```python
from build123d import *

# Parameters (mm, degrees)
F0_R      = 12.5
F0_R_2    = 2.2070756532
F1_DEPTH  = 16
F2_W      = 30
F2_H      = 115
F2_W_2    = 115
F2_H_2    = 30
F3_DEPTH  = 30
F5_W      = 47.7929243468
F5_H      = 100
F5_W_2    = 30
F5_W_3    = 37.2070756532
F6_DEPTH  = 5
F7_W      = 115
F7_H      = 100
F8_DEPTH  = 5
F10_W     = 115
F10_H     = 100
F11_DEPTH = 5
F9_W      = 30
F9_H      = 100
F9_W_2    = 37.2870707512
F13_DEPTH = 5
F14_D     = 8
F14_DEPTH = 35.001


with BuildPart() as f1:
    # F0 (on Front) → F1 (new body)
    with BuildSketch(Plane.XZ):
        with BuildLine():
            Line((-699.9135494232, 64.4235223532), (-699.9135494232, -435.5764776468))
            Line((-699.9135494232, -435.5764776468), (-70.5764776468, -435.5764776468))
            Line((-70.5764776468, -435.5764776468), (0.0864505768, -364.9135494232))
            Line((0.0864505768, -364.9135494232), (0.0864505768, -2.20538188))
            ThreePointArc((0.0864505768, -2.20538188), (-2.2070756532, 0), (0.0864505768, 2.20538188))
            Line((0.0864505768, 2.20538188), (0.0864505768, 64.4235223532))
            Line((0.0864505768, 64.4235223532), (-149.9135494232, 64.4235223532))
            Line((-149.9135494232, 64.4235223532), (-149.9135494232, 49.4235223532))
            Line((-149.9135494232, 49.4235223532), (-319.9135494232, 49.4235223532))
            Line((-319.9135494232, 49.4235223532), (-319.9135494232, 64.4235223532))
            Line((-319.9135494232, 64.4235223532), (-699.9135494232, 64.4235223532))
        make_face()
        with Locations((-599.9135494232, -355.5764776468)):
            Circle(F0_R, mode=Mode.SUBTRACT)
        with Locations((-594.9135494232, -320.5764776468)):
            Circle(F0_R_2, mode=Mode.SUBTRACT)
        with Locations((-509.9135494232, -320.5764776468)):
            Circle(F0_R_2, mode=Mode.SUBTRACT)
        with Locations((-594.9135494232, -250.5764776468)):
            Circle(F0_R_2, mode=Mode.SUBTRACT)
        with Locations((-509.9135494232, -250.5764776468)):
            Circle(F0_R_2, mode=Mode.SUBTRACT)
        with Locations((-99.9135494232, -320.5764776468)):
            Circle(F0_R_2, mode=Mode.SUBTRACT)
        with Locations((-19.9135494232, -355.5764776468)):
            Circle(F0_R, mode=Mode.SUBTRACT)
        with Locations((-14.9135494232, -320.5764776468)):
            Circle(F0_R_2, mode=Mode.SUBTRACT)
        with Locations((-99.9135494232, -250.5764776468)):
            Circle(F0_R_2, mode=Mode.SUBTRACT)
        with Locations((-14.9135494232, -250.5764776468)):
            Circle(F0_R_2, mode=Mode.SUBTRACT)
        with Locations((-399.9135494232, -160.5764776468)):
            Circle(F0_R_2, mode=Mode.SUBTRACT)
        with Locations((-400.6345868111, -90.5764776468)):
            Circle(F0_R_2, mode=Mode.SUBTRACT)
        with Locations((-594.9135494232, -25.5764776468)):
            Circle(F0_R_2, mode=Mode.SUBTRACT)
        with Locations((-599.9135494232, 44.4235223532)):
            Circle(F0_R, mode=Mode.SUBTRACT)
        with Locations((-509.9135494232, -25.5764776468)):
            Circle(F0_R_2, mode=Mode.SUBTRACT)
        with Locations((-509.9135494232, 44.4235223532)):
            Circle(F0_R_2, mode=Mode.SUBTRACT)
        with Locations((-314.9135494232, -160.5764776468)):
            Circle(F0_R_2, mode=Mode.SUBTRACT)
        with Locations((-315.6345868111, -90.5764776468)):
            Circle(F0_R_2, mode=Mode.SUBTRACT)
        with Locations((-19.9135494232, 44.4235223532)):
            Circle(F0_R, mode=Mode.SUBTRACT)
        with BuildLine():
            ThreePointArc((0.0864505768, 2.20538188), (-2.2070756532, 0), (0.0864505768, -2.20538188))
            Line((0.0864505768, -2.20538188), (0.0864505768, 2.20538188))
        make_face()
        with BuildLine():
            Line((0.0864505768, 2.20538188), (0.0864505768, -2.20538188))
            ThreePointArc((0.0864505768, -2.20538188), (1.5909094729, -1.5297679523), (2.2070756532, 0))
            ThreePointArc((2.2070756532, 0), (1.5909094729, 1.5297679523), (0.0864505768, 2.20538188))
        make_face()
    extrude(amount=-F1_DEPTH)

    # F2 (on Front) → F3 (join)
    with BuildSketch(Plane.XZ):
        with Locations((-547.1206250764, -280.2835533)):
            Rectangle(F2_W, F2_H)
        with Locations((-355.6849062443, -120.1901584864)):
            Rectangle(F2_W, F2_H)
        with Locations((-547.2006201744, 6.2219314277)):
            Rectangle(F2_W, F2_H)
        with Locations((-62.3018592596, -282.930508256)):
            Rectangle(F2_W, F2_H)
        with Locations((-59.2683969438, -3.8263390213)):
            Rectangle(F2_W_2, F2_H_2)
    extrude(amount=F3_DEPTH)

    # F5 (on face) → F6 (join)
    with BuildSketch(Plane.XZ.offset(30)):
        with Locations((-586.0170872498, -285.5764776468)):
            Rectangle(F5_W, F5_H)
        with Locations((-547.1206250764, -285.5764776468)):
            Rectangle(F5_W_2, F5_H)
        with Locations((-513.5170872498, -285.5764776468)):
            Rectangle(F5_W_3, F5_H)
    extrude(amount=F6_DEPTH)

    # F7 (on face) → F8 (join)
    with BuildSketch(Plane.XZ.offset(30)):
        with Locations((-57.4135494232, -282.930508256)):
            Rectangle(F7_W, F7_H)
    extrude(amount=F8_DEPTH)

    # F10 (on face) → F11 (join)
    with BuildSketch(Plane.XZ.offset(30)):
        with Locations((-358.1345868111, -124.6901584864)):
            Rectangle(F10_W, F10_H)
    extrude(amount=F11_DEPTH)

    # F9 (on face) → F13 (join)
    with BuildSketch(Plane.XZ.offset(30)):
        Polygon((-562.2006201744, -40.5764776468), (-562.2006201744, 59.4235223532), (-574.9135494232, 59.4235223532), (-574.9135494232, 24.4235223532), (-609.9135494232, 24.4235223532), (-609.9135494232, -40.5764776468), align=None)
        with Locations((-547.2006201744, 9.4235223532)):
            Rectangle(F9_W, F9_H)
        with Locations((-513.5570847988, 9.4235223532)):
            Rectangle(F9_W_2, F9_H)
    extrude(amount=F13_DEPTH)

    # F14 (through all, one way)
    with BuildSketch(Plane(origin=(0, 0, 0), x_dir=(1, 0, 0), z_dir=(0, 1, 0))):
        with Locations((-594.9135494232, 250.5764776468), (-594.9135494232, 320.5764776468), (-509.9135494232, 320.5764776468), (-509.9135494232, 250.5764776468), (-400.6345868111, 90.5764776468), (-315.6345868111, 90.5764776468), (-399.9135494232, 160.5764776468), (-314.9135494232, 160.5764776468), (-594.9135494232, 25.5764776468), (-509.9135494232, 25.5764776468), (-509.9135494232, -44.4235223532), (-99.9135494232, 320.5764776468), (-99.9135494232, 250.5764776468), (-14.9135494232, 320.5764776468), (-14.9135494232, 250.5764776468)):
            Circle(F14_D / 2)
    extrude(amount=-F14_DEPTH, mode=Mode.SUBTRACT)


solid = f1.part
```
CAD build for the part. Positions are in the model's coordinates, mm. A direction names the side the tool comes from. Round coordinates to 2 decimals unless told otherwise and drop trailing zeros. Order: outer loops, then holes, each group sorted by start corner. A loop starts at its lowest first (then second) coordinate and runs counter-clockwise, first axis right, second up. Notation, with made-up numbers: (31, -37) - (55, -37) arc R35 cw to (55, -1) - close; hole circle Ø7 at (75, 77). An arc over 180 degrees is marked (long way). Use CSV: the item, a comma, the result in double quotes. Start each with the question number.
1) Saw through at D-D (z = -399). List the corners of the cut face in (x, y).
2) Wall check: L1, parallel to Y at x = -334, z = -132.5; L2, parallel to X at y = -15, z = -16; L3, parallel to Y at x = -433.5, z = -344. Give the ranges that are in metal, low to high. Write a range as [from, to].
3) Pin check, flat tips, straight feed: pin 1 Ø5 at (x, z) = (-400.63, -90.58) entering from -Y; pin 2 Ø5.5 at (x, y) = (-594, -32) entering from +Z; pin 3 Ø5.5 at (y, z) = (-32.5, -294) entering from -X. Stop position of each tip, or through.
4) Saw through at C-C (x = -205). List the corners of the cut face in (y, z).
5) Saw through at A-A (y = -7). List the corners of the cut face in (x, z).
6) Two-plate mould, pull along Y, no slides. Class faces 1 (the flat face through (-547, -15, -51.278)), 2 (the flat face through (-359, -35, -124)), 3 (the flat face through (-24, -30, -282)): pulls with the +Y half, pulls with the -Y half, needs draft (parallel to the pull), parting line crosses it, or undercut.
7) Tool access for faces 4 (the flat face through (-60, -30, -4)), 5 (the flat face through (-319.914, 8, 57)), 6 (the flat face through (-547, -15, 63.722)), 7 (the flat face through (-63, -15, -225.431)), 8 (the flat face through (-1.768, -15, -4)): list every direction of +Z, -Z, +X, -X, +Y, -Y with a clear straight run to the whole face (end or side of a thin tool).
8) Saw through at B-B (z = -105.5). List the corners of the cut face in (x, y).
Values follow:
1,outline,"(-699.91, 0) - (-34, 0) - (-34, 16) - (-699.91, 16) - close"
2,L1,"y = [-35, -30], [0, 16]"
2,L2,"x = [-562.2, -532.2], [-116.77, -1.77]"
2,L3,"y = [0, 16]"
3,pin 1,"stops at y = 0"
3,pin 2,"stops at z = 24.42"
3,pin 3,"stops at x = -609.91"
4,outline,"(0, -435.58) - (16, -435.58) - (16, 49.42) - (0, 49.42) - close"
5,outline,"(-562.2, -51.28) - (-532.2, -51.28) - (-532.2, 63.72) - (-562.2, 63.72) - close; (-562.12, -337.78) - (-532.12, -337.78) - (-532.12, -222.78) - (-562.12, -222.78) - close; (-370.68, -177.69) - (-340.68, -177.69) - (-340.68, -62.69) - (-370.68, -62.69) - close; (-116.77, -18.83) - (-1.77, -18.83) - (-1.77, 11.17) - (-116.77, 11.17) - close; (-77.3, -340.43) - (-47.3, -340.43) - (-47.3, -225.43) - (-77.3, -225.43) - close"
6,face 1,"needs draft"
6,face 2,"pulls with the -Y half"
6,face 3,"undercut"
7,face 4,"+Z, +X, -Y"
7,face 5,"+Z, +Y, -Y"
7,face 6,"+Z, +X, -X, -Y"
7,face 7,"+X, -Y"
7,face 8,"+Z, -Z, +X, -Y"
8,outline,"(-699.91, 0) - (-370.68, 0) - (-370.68, -30) - (-415.63, -30) - (-415.63, -35) - (-300.63, -35) - (-300.63, -30) - (-340.68, -30) - (-340.68, 0) - (0.09, 0) - (0.09, 16) - (-699.91, 16) - close"
